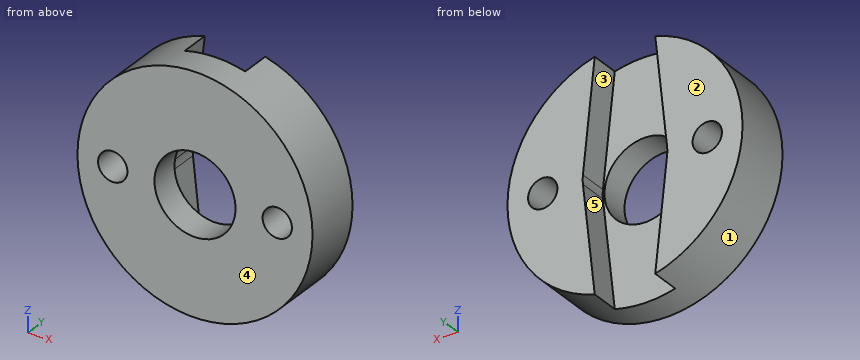
```python
from build123d import *

# Parameters (mm, degrees)
SKETCH1_R                       = 10
BOSS_EXTRUDE1_DEPTH             = 5
TAP_DRILL_FOR_M3X0_5_TAP1_D     = 2.5
TAP_DRILL_FOR_M3X0_5_TAP1_DEPTH = 38.1
CIRPATTERN1_COUNT               = 4
F_14_0_182_DIAMETER_HOLE1_D     = 6.899999916
CUT_EXTRUDE3_DEPTH              = 2.5


with BuildPart() as part:
    # Sketch1 → Boss-Extrude1 (new body)
    with BuildSketch(Plane(origin=(0, 0, 0), x_dir=(1, 0, 0), z_dir=(0, 1, 0))):
        Circle(SKETCH1_R)
    extrude(amount=BOSS_EXTRUDE1_DEPTH)

    # Tap Drill for M3x0.5 Tap1
    with Locations(Plane(origin=(0, 5, 0), x_dir=(1, 0, 0), z_dir=(0, 1, 0))):
        with Locations((7, 0)):
            tap_drill_for_m3x0_5_tap1 = Hole(TAP_DRILL_FOR_M3X0_5_TAP1_D / 2, depth=TAP_DRILL_FOR_M3X0_5_TAP1_DEPTH)

    # CirPattern1: Tap Drill for M3x0.5 Tap1 ×4 about axis, 2 skipped
    cirpattern1_axis = Axis((0, 5, 0), (0, -1, 0))
    add([tap_drill_for_m3x0_5_tap1.rotate(cirpattern1_axis, i * 360 / CIRPATTERN1_COUNT) for i in range(1, CIRPATTERN1_COUNT) if i not in (1, 3)], mode=Mode.SUBTRACT)

    # #14 (0.182) Diameter Hole1 (through all)
    with Locations(Plane(origin=(0, 5, 0), x_dir=(1, 0, 0), z_dir=(0, 1, 0))):
        with Locations((0, 0)):
            Hole(F_14_0_182_DIAMETER_HOLE1_D / 2)

    # Sketch10 → Cut-Extrude3 (cut)
    with BuildSketch(Plane(origin=(0, 5, 0), x_dir=(1, 0, 0), z_dir=(0, 1, 0))):
        with BuildLine():
            Line((-3.57904225, 0.387887324), (-2.057949293, 14.423035211))
            ThreePointArc((-2.057949293, 14.423035211), (0, 16.27), (2.057949293, 14.423035211))
            Line((2.057949293, 14.423035211), (3.57904225, 0.387887324))
            ThreePointArc((3.57904225, 0.387887324), (3.6, 0), (3.57904225, -0.387887324))
            Line((3.57904225, -0.387887324), (2.057949293, -14.423035211))
            ThreePointArc((2.057949293, -14.423035211), (0, -16.27), (-2.057949293, -14.423035211))
            Line((-2.057949293, -14.423035211), (-3.57904225, -0.387887324))
            ThreePointArc((-3.57904225, -0.387887324), (-3.6, 0), (-3.57904225, 0.387887324))
        make_face()
    extrude(amount=-CUT_EXTRUDE3_DEPTH, mode=Mode.SUBTRACT)


solid = part.part
```
Source: CAD feature listing. Evaluate the final solid. Frame: model axes, mm. Face numbers are marked on the shaded views. A direction names the side the tool comes from. Give positions to 0.01 mm unless a question says otherwise; leave off trailing zeros. Order: outer loops, then holes, each group sorted by start corner. A loop starts at its lowest first (then second) coordinate and runs counter-clockwise, first axis right, second up.
(1) Access query for the marked faces 4 and 5. Directions: +Z, -Z, +X, -X, +Y, -Y. A direction counts if a zero-diameter tool reaches every point of the face in a straight line with its end or side. Return the directions, or none.
(2) Pull-direction query (Z, two-part tool) for the marked faces 1, 2 and 3; classes: +Z half, -Z half, draft (parallel to the pull), parting line (faces both ways), or undercut.
(3) Section query D-D (z = 7.75). Return the cut outline in (x, y).
(4) Section query B-B (z = 0). Return the cut outline in (x, y).
(5) Section query A-A (y = 3.1). Return the cut outline in (x, z), plus the area to 3 significant figures.
(6) Material intervals for line 1 along Z through (x, y) = (0, 1.35); line 2 along X through (y, z) = (2.9, 4.25); line 3 along Z through (x, y) = (7, 2.1), sorted ascending.
(7) Section query C-C (x = 0). Return the cut outline in (y, z), plus the area to 4 significant figures.
(8) Contact query for a flat-ended pin moving along its axis: P1, Ø1, axis at y = 4, z = -7, coming from the -X side. Output: stop coordinate, or through.
Outcome:
1. face 4: +Z, -Z, +X, -X, -Y
1. face 5: +Y
2. face 1: parting line
2. face 2: draft
2. face 3: undercut
3. outline: (-6.32, 0) - (6.32, 0) - (6.32, 5) - (2.78, 5) - (2.78, 2.5) - (-2.78, 2.5) - (-2.78, 5) - (-6.32, 5) - close
4. outline: (-10, 0) - (-8.25, 0) - (-8.25, 5) - (-10, 5) - close; (-5.75, 0) - (-3.45, 0) - (-3.45, 2.5) - (-3.6, 2.5) - (-3.6, 5) - (-5.75, 5) - close; (3.45, 0) - (5.75, 0) - (5.75, 5) - (3.6, 5) - (3.6, 2.5) - (3.45, 2.5) - close; (8.25, 0) - (10, 0) - (10, 5) - (8.25, 5) - close
5. outline: (-3.58, -0.39) arc R3.6 cw to (-3.58, 0.39) - (-2.57, 9.66) arc R10 ccw to (-2.57, -9.66) - close; (2.57, -9.66) arc R10 ccw to (2.57, 9.66) - (3.58, 0.39) arc R3.6 cw to (3.58, -0.39) - close; hole circle Ø2.5 at (-7, 0); hole circle Ø2.5 at (7, 0)
5. area: 182 mm2
6. line 1: z = -10 to -3.45, 3.45 to 10
6. line 2: x = -9.05 to -3.16, 3.16 to 9.05
6. line 3: z = -7.14 to -1.25, 1.25 to 7.14
7. outline: (0, -10) - (2.5, -10) - (2.5, -3.45) - (0, -3.45) - close; (0, 3.45) - (2.5, 3.45) - (2.5, 10) - (0, 10) - close
7. area: 32.75 mm2
8. P1: stops at x = -7.6
